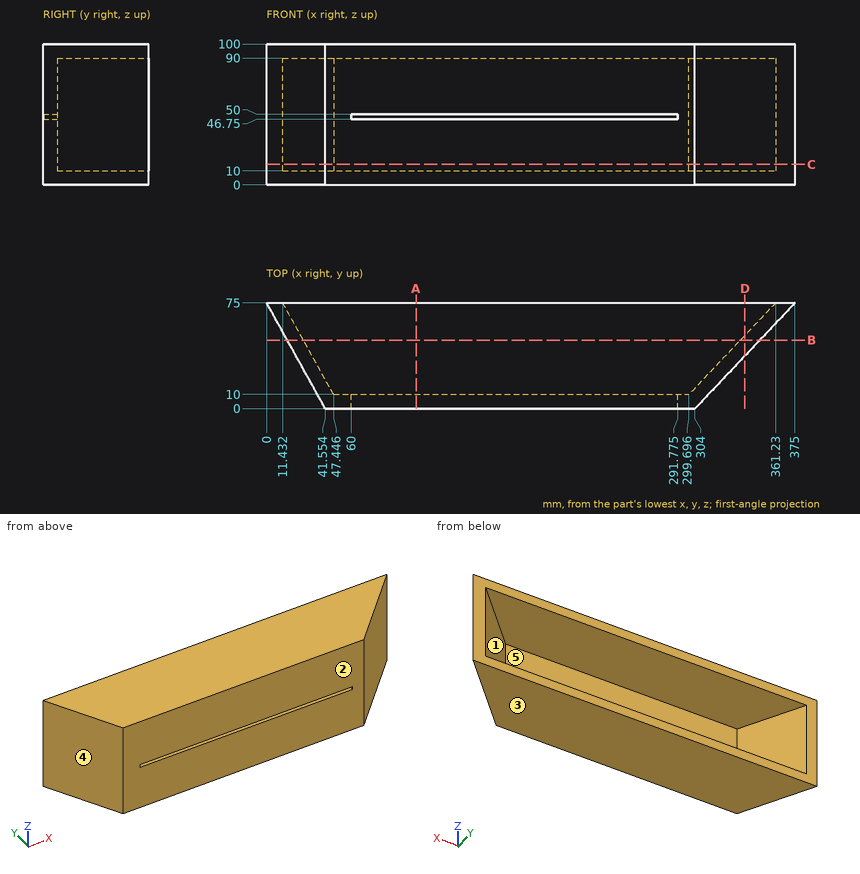
Answer from the drawing. Dimensions are ordinates in mm from the lowest x, y and z of the part. A direction names the side the tool comes from. Give positions to 0.01 mm unless a question says otherwise; leave off trailing zeros. Order: outer loops, then holes, each group sorted by start corner. A loop starts at its lowest first (then second) coordinate and runs counter-clockwise, first axis right, second up.
(1) Find section D-D (x = 339.5). Give the vertices of the cut face in (y, z) (1 decimal).
(2) Straight lines are drawn through the part: L1, parallel to Z at x = 158, y = 17; L2, parallel to X at y = 25.5, z = 41 (1 decimal); L3, parallel to Y at x = 227.5, z = 20. For each, find the intervals that lie inside material, in ascending order.
(3) Given pin 1 (4 mm diameter, centred on y = 40.5, z = 23.5, fed in from +X) (1 decimal); pin 2 (10 mm diameter, centred on y = 11, z = 36.5, fed in from +X) (1 decimal); pin 3 (1 mm diameter, centred on y = 7.5, z = 48.5, fed in from -X), each flat-ended and moving along its own axis, determine where each tip first touches the part or whether it passes through.
(4) For a pull along Z with two mould halves and no side action, classify the marked faces 3, 4 and 5 as released by +Z, released by -Z, zero draft, split by the parting line, or undercut.
(5) Find section A-A (x = 106). Give the vertices of the cut face in (y, z).
(6) Find section B-B (y = 48.5). Give the vertices of the cut face in (x, z) (1 decimal), plus the area to 3 significant figures.
(7) Find section C-C (z = 14.5). Give the vertices of the cut face in (x, y) (1 decimal).
(8) For the marked faces 1 and 2, determine the directions among +Z, -Z, +X, -X, +Y, -Y from which every point of the face is accessible in a straight line to the end or side of a thin tool.
Result sheet:
1. outline: (37.5, 0) - (75, 0) - (75, 10) - (52, 10) - (52, 90) - (75, 90) - (75, 100) - (37.5, 100) - close
2. L1: z = 0 to 10, 90 to 100
2. L2: x = 27.4 to 38.9, 314.4 to 328.1
2. L3: y = 0 to 10
3. pin 1: stops at x = 344.2
3. pin 2: stops at x = 319.1
3. pin 3: stops at x = 37.12
4. face 3: released by -Z
4. face 4: zero draft
4. face 5: undercut
5. outline: (0, 0) - (75, 0) - (75, 10) - (10, 10) - (10, 46.75) - (0, 46.75) - close; (0, 50) - (10, 50) - (10, 90) - (75, 90) - (75, 100) - (0, 100) - close
6. outline: (14.7, 0) - (349.9, 0) - (349.9, 100) - (14.7, 100) - close; hole (26.1, 10) - (336.1, 10) - (336.1, 90) - (26.1, 90) - close
6. area: 8,720 mm2
7. outline: (0, 75) - (41.6, 0) - (304, 0) - (375, 75) - (361.2, 75) - (299.7, 10) - (47.4, 10) - (11.4, 75) - close
8. face 1: +Y
8. face 2: +Z, -Z, +X, -X, -Y
